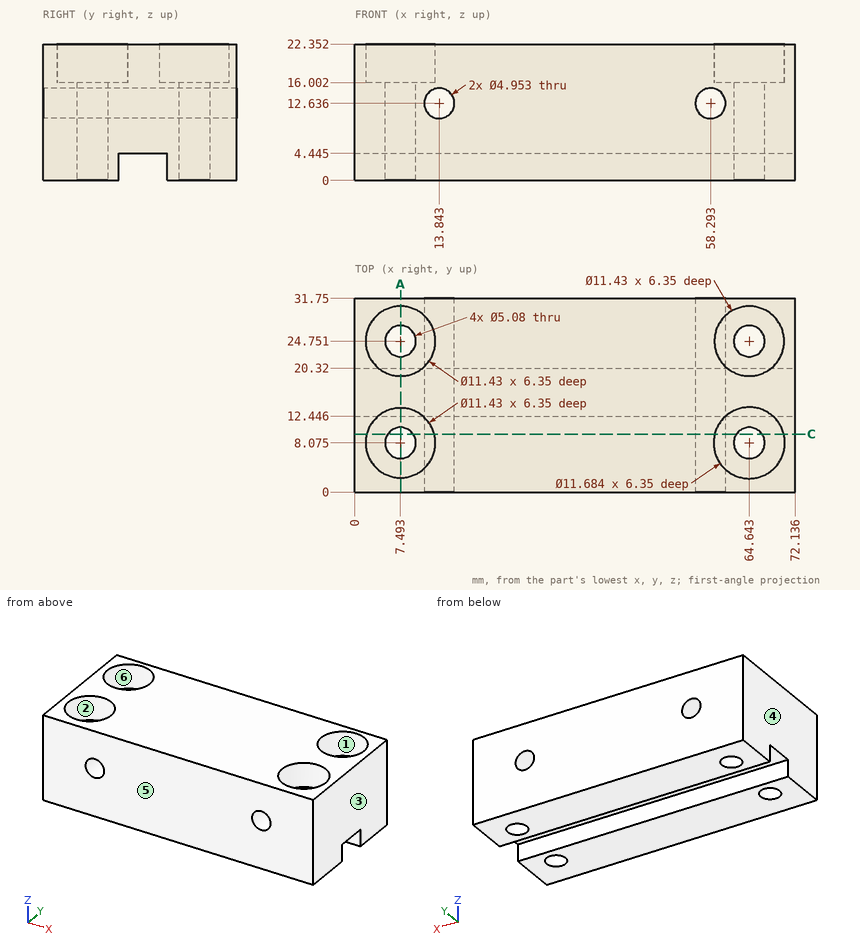
Could you check a few things on this drawing? It's one solid part, dimensions in mm from its lowest x, y, z. A direction names the side the tool comes from. Coordinates: 2 decimals unless noted, no trailing zeros. Write each loop counter-clockwise with the first axis right and the second up, starting at its lowest first coordinate (ties: lowest second). Pieces come first, ordered by that corner, then holes. Notation, with made-up numbers: (27, 6) - (62, 6) arc R18 ccw to (62, 11) - close; hole circle Ø4 at (61.5, 47.5). An arc over 180 degrees is marked (long way). Write item = value, one per line.
1) Suppose I cut it at A-A on x = 7.5. State how many separate pieces and enclosed holes the cut face has, plus the area to 3 significant figures.
Result set:
separate_pieces = 3
enclosed_holes = 0
area = 367 mm2
2) Will these pins go through, and if not, where does the flat tip stop? pin 1 Ø3.5 at (x, y) = (8.5, 9) entering from +Z; pin 2 Ø2.5 at (x, y) = (32.5, 18) entering from -Z (1 decimal).
Result set:
pin_1 = 16
pin_2 = 4.4
3) For the marked faces 5 and 6, which set-ups out of +Z, -Z, +X, -X, +Y, -Y let a thin tool reach every point of the face, with its end or its side?
Result set:
face_5 = +Z, -Z, +X, -X, -Y
face_6 = +Z
4) We'd pull the mould along X, two halves only. Please class the marked faces 1, 2, 3 and 4: +X half, -X half, draft (parallel to the pull), parting line (faces both ways), or undercut.
Result set:
face_1 = undercut
face_2 = undercut
face_3 = +X half
face_4 = -X half
5) Please list where these lines run through material, in increasing order: line 1 (X direction, y = 29, z = 12.5) (1 decimal); line 2 (X direction, y = 7.5, z = 17.75) (1 decimal); line 3 (X direction, y = 26, z = 14.5) (1 decimal). Write a range as [from, to].
Result set:
line_1 = [0, 11.4], [16.3, 55.8], [60.8, 72.1]
line_2 = [0, 1.8], [13.2, 58.8], [70.5, 72.1]
line_3 = [0, 5.3], [9.7, 12.2], [15.5, 56.7], [59.9, 62.4], [66.9, 72.1]
6) Suppose I cut it at C-C on y = 9.5. Please give me the cut outline in (x, z) (1 decimal), plus the area to 3 significant figures.
Result set:
outline = (0, 0) - (5.4, 0) - (5.4, 16) - (2, 16) - (2, 22.4) - (0, 22.4) - close; (9.6, 0) - (62.5, 0) - (62.5, 16) - (59, 16) - (59, 22.4) - (13, 22.4) - (13, 16) - (9.6, 16) - close; (66.7, 0) - (72.1, 0) - (72.1, 22.4) - (70.3, 22.4) - (70.3, 16) - (66.7, 16) - close; hole circle Ø5 at (13.8, 12.6); hole circle Ø5 at (58.3, 12.6)
area = 1,300 mm2
